from build123d import *

# Parameters (mm, degrees)
SALIENTE_EXTRUIR1_DEPTH = 3
REDONDEO1_R             = 0.25


with BuildPart() as part:
    # Croquis1 → Saliente-Extruir1 (new body)
    with BuildSketch(Plane(origin=(0, 0, 0), x_dir=(1, 0, 0), z_dir=(0, 1, 0))):
        with BuildLine():
            Line((0, 3.55), (0, -3.55))
            ThreePointArc((0, -3.55), (0.292893219, -4.257106781), (1, -4.55))
            Line((1, -4.55), (12, -4.55))
            ThreePointArc((12, -4.55), (12.707106781, -4.257106781), (13, -3.55))
            Line((13, -3.55), (13, -1.55))
            Line((13, -1.55), (8, -1.55))
            Line((8, -1.55), (8, 1.55))
            Line((8, 1.55), (13, 1.55))
            Line((13, 1.55), (13, 3.55))
            ThreePointArc((13, 3.55), (12.707106781, 4.257106781), (12, 4.55))
            Line((12, 4.55), (1, 4.55))
            ThreePointArc((1, 4.55), (0.292893219, 4.257106781), (0, 3.55))
        make_face()
    extrude(amount=SALIENTE_EXTRUIR1_DEPTH)

    # Redondeo1
    redondeo1_edges = [part.edges().sort_by_distance(p)[0] for p in [
        (13, 1.5, -1.55),
        (8, 1.5, -1.55),
        (8, 1.5, 1.55),
        (13, 1.5, 1.55),
    ]]
    fillet(redondeo1_edges, radius=REDONDEO1_R)


solid = part.part
Verification items for the finished model (mm, model axes). A direction names the side the tool comes from. Give positions to 0.01 mm unless a question says otherwise; leave off trailing zeros. Order: outer loops, then holes, each group sorted by start corner. A loop starts at its lowest first (then second) coordinate and runs counter-clockwise, first axis right, second up. Notation, with made-up numbers: M 29,51.5 L 47,51.5 A27 ccw 47,76.5 Z; hole C 5.25,83.5 d8. An arc over 180 degrees is marked long. Answer as a JSON object with one key per item and string values. Group by question number.
1) Cross-section at B-B (y = 1.3). Enter the section's corners in (x, z).
2) Access from +Z, -Z, +X, -X, +Y, -Y to the whole of each face (thin tool, end or side, straight path). Record for faces 5 (the face through (0.285, 1.479, 4.249)), 6 (the face through (11, 1, 1.55)).
3) Mould release check, pull along Z, two halves, no side actions. Record for faces 1 (the face through (6, 3, 0)), 2 (the face through (7, 1, -4.55)), 3 (the face through (8, 1, 0)), 4 (the face through (10, 1, -1.55)): released by +Z, released by -Z, zero draft, split by the parting line, or undercut.
4) Cross-section at A-A (x = 9.75). Enter the section's corners in (y, z).
5) Scan lines: line 1 along Z through (x, y) = (10, 2.95); line 2 along X through (y, z) = (2.8, 0.25); line 3 along Z through (x, y) = (12.25, 1.15). Record each from-to range of solid material in increasing order. Write a range as [from, to].
6) Cross-section at C-C (z = -1). Enter the section's corners in (x, y).
Result sheet:
{
 "1": {"outline": "M 0,-3.55 A1 ccw 1,-4.55 L 12,-4.55 A1 ccw 13,-3.55 L 13,-1.8 A0.25 ccw 12.75,-1.55 L 8.25,-1.55 A0.25 cw 8,-1.3 L 8,1.3 A0.25 cw 8.25,1.55 L 12.75,1.55 A0.25 ccw 13,1.8 L 13,3.55 A1 ccw 12,4.55 L 1,4.55 A1 ccw 0,3.55 Z"},
 "2": {"face 5": "+Z, -X, +Y, -Y", "face 6": "+X, +Y, -Y"},
 "3": {"face 1": "zero draft", "face 2": "released by -Z", "face 3": "undercut", "face 4": "undercut"},
 "4": {"outline": "M 0,-4.55 L 3,-4.55 L 3,-1.55 L 0,-1.55 Z; M 0,1.55 L 3,1.55 L 3,4.55 L 0,4.55 Z"},
 "5": {"line 1": "z = [-4.55, -1.55], [1.55, 4.55]", "line 2": "x = [0, 8]", "line 3": "z = [-4.52, -1.55], [1.55, 4.52]"},
 "6": {"outline": "M 0,0 L 8,0 L 8,3 L 0,3 Z"}
}
